from build123d import *

# Parameters (mm, degrees)
SKETCH_1_W          = 20
SKETCH_1_H          = 32.8
EXTRUDE_1_DEPTH     = 4
CUT_EXTRUDE_1_DEPTH = 1.6
SKETCH_4_R          = 2
CUT_EXTRUDE_2_DEPTH = 1.5
SKETCH_4_3_R        = 1.25
CUT_EXTRUDE_3_DEPTH = 39.624344655
SKETCH_5_W          = 20
SKETCH_5_H          = 6.2
EXTRUDE_4_DEPTH     = 2
EXTRUDE_START       = 2
SKETCH_5_6_W        = 20
SKETCH_5_6_H        = 4
EXTRUDE_5_DEPTH     = 5
SKETCH_6_R          = 1.25
CUT_EXTRUDE_4_DEPTH = 39.913750783
SKETCH_6_3_R        = 2
CUT_EXTRUDE_5_DEPTH = 1.5


with BuildPart() as part:
    # 草图1 → 凸台-拉伸1 (new body)
    with BuildSketch(Plane(origin=(0, 0, 0), x_dir=(1, 0, 0), z_dir=(0, 1, 0))):
        with Locations((10, -16.4)):
            Rectangle(SKETCH_1_W, SKETCH_1_H)
    extrude(amount=EXTRUDE_1_DEPTH)

    # 草图3 → 切除-拉伸1 (cut)
    with BuildSketch(Plane(origin=(0, 4, 0), x_dir=(-1, 0, 0), z_dir=(0, 1, 0))):
        with BuildLine():
            Line((-12.8, 13.543428629), (-12.095952788, 2.219685343))
            ThreePointArc((-12.095952788, 2.219685343), (-10, 0.25), (-7.904047212, 2.219685343))
            Line((-7.904047212, 2.219685343), (-7.2, 13.543428629))
            ThreePointArc((-7.2, 13.543428629), (-6, 16.4), (-7.2, 19.256571371))
            Line((-7.2, 19.256571371), (-7.904047212, 30.580314657))
            ThreePointArc((-7.904047212, 30.580314657), (-10, 32.55), (-12.095952788, 30.580314657))
            Line((-12.095952788, 30.580314657), (-12.8, 19.256571371))
            ThreePointArc((-12.8, 19.256571371), (-14, 16.4), (-12.8, 13.543428629))
        make_face()
    extrude(amount=-CUT_EXTRUDE_1_DEPTH, mode=Mode.SUBTRACT)

    # 草图4 → 切除-拉伸2 (cut)
    with BuildSketch(Plane.XZ):
        with Locations(Location((4, 4, 0), (0, 0, 270))):
            Circle(SKETCH_4_R)
        with Locations(Location((4, 28.8, 0), (0, 0, 270))):
            Circle(SKETCH_4_R)
        with Locations(Location((16, 28.8, 0), (0, 0, 270))):
            Circle(SKETCH_4_R)
        with Locations(Location((16, 4, 0), (0, 0, 270))):
            Circle(SKETCH_4_R)
    extrude(amount=-CUT_EXTRUDE_2_DEPTH, mode=Mode.SUBTRACT)

    # 草图4<3> → 切除-拉伸3 (cut, through all)
    with BuildSketch(Plane.XZ):
        with Locations(Location((4, 4, 0), (0, 0, 270))):
            Circle(SKETCH_4_3_R)
        with Locations(Location((4, 28.8, 0), (0, 0, 270))):
            Circle(SKETCH_4_3_R)
        with Locations(Location((16, 4, 0), (0, 0, 270))):
            Circle(SKETCH_4_3_R)
        with Locations(Location((16, 28.8, 0), (0, 0, 270))):
            Circle(SKETCH_4_3_R)
    extrude(amount=-CUT_EXTRUDE_3_DEPTH, mode=Mode.SUBTRACT)

    # 草图5 → 凸台-拉伸4 (add)
    with BuildSketch(Plane(origin=(0, 0, 0), x_dir=(-1, 0, 0), z_dir=(0, 0, -1))):
        with Locations((-10, 3.1)):
            Rectangle(SKETCH_5_W, SKETCH_5_H)
    extrude(amount=EXTRUDE_4_DEPTH)

    # 草图5<6> → 凸台-拉伸5 (add)
    with BuildSketch(Plane(origin=(0, 0, 0), x_dir=(-1, 0, 0), z_dir=(0, 0, -1)).offset(EXTRUDE_START)):
        with Locations((-10, 2)):
            Rectangle(SKETCH_5_6_W, SKETCH_5_6_H)
    extrude(amount=EXTRUDE_5_DEPTH)

    # 草图6 → 切除-拉伸4 (cut, through all)
    with BuildSketch(Plane.XZ):
        with Locations(Location((4, -4.5, 0), (0, 0, 270))):
            Circle(SKETCH_6_R)
        with Locations(Location((16, -4.5, 0), (0, 0, 270))):
            Circle(SKETCH_6_R)
    extrude(amount=-CUT_EXTRUDE_4_DEPTH, mode=Mode.SUBTRACT)

    # 草图6<3> → 切除-拉伸5 (cut)
    with BuildSketch(Plane.XZ):
        with Locations(Location((4, -4.5, 0), (0, 0, 270))):
            Circle(SKETCH_6_3_R)
        with Locations(Location((16, -4.5, 0), (0, 0, 270))):
            Circle(SKETCH_6_3_R)
    extrude(amount=-CUT_EXTRUDE_5_DEPTH, mode=Mode.SUBTRACT)


solid = part.part
Check sheet for the modelled part. Datum: model origin and axes. Units: mm. A direction names the side the tool comes from. Round coordinates to 2 decimals unless told otherwise and drop trailing zeros. Order: outer loops, then holes, each group sorted by start corner. A loop starts at its lowest first (then second) coordinate and runs counter-clockwise, first axis right, second up.
Q1. Cross-section at D-D, the plane x = 10. Enter the section's corners in (y, z).
Filled sheet:
outline: (0, -7) - (4, -7) - (4, -2) - (6.2, -2) - (6.2, 0) - (4, 0) - (4, 0.25) - (2.4, 0.25) - (2.4, 32.55) - (4, 32.55) - (4, 32.8) - (0, 32.8) - close
Q2. Cross-section at A-A, the plane x = 16. Give the number of separate pieces and of enclosed holes in the cut face, plus the area to 3 significant figures.
Filled sheet:
separate pieces: 4
enclosed holes: 0
area: 127 mm2
Q3. Cross-section at C-C, the plane y = 3. Enter the section's corners in (x, z), plus the area to 3 significant figures.
Filled sheet:
outline: (0, -7) - (20, -7) - (20, 32.8) - (0, 32.8) - close; hole circle Ø2.5 at (4, -4.5); hole circle Ø2.5 at (4, 4); hole circle Ø2.5 at (4, 28.8); hole (7.2, 13.54) - (7.9, 2.22) arc R2.1 ccw to (12.1, 2.22) - (12.8, 13.54) arc R4 ccw to (12.8, 19.26) - (12.1, 30.58) arc R2.1 ccw to (7.9, 30.58) - (7.2, 19.26) arc R4 ccw to start; hole circle Ø2.5 at (16, -4.5); hole circle Ø2.5 at (16, 4); hole circle Ø2.5 at (16, 28.8)
area: 601 mm2
Q4. Scan lines: L1, parallel to X at y = 0.6, z = 28.8; L2, parallel to Z at x = 3.75, y = 3; L3, parallel to Z at x = 16.5, y = 2. Record each from-to range of solid material in increasing order.
Filled sheet:
L1: x = 0 to 2, 6 to 14, 18 to 20
L2: z = -7 to -5.72, -3.28 to 2.78, 5.22 to 27.58, 30.02 to 32.8
L3: z = -7 to -5.65, -3.35 to 2.85, 5.15 to 27.65, 29.95 to 32.8
Q5. Depth check by flat-ended pin: P1, Ø6.5, axis at x = 16, z = 28.8, coming from the +Y side; P2, Ø3.5, axis at x = 4, z = 28.8, coming from the -Y side; P3, Ø2, axis at x = 10.5, z = 12.5, coming from the +Y side. Enter the tip coordinate at first touch or a pass-through.
Filled sheet:
P1: stops at y = 4
P2: stops at y = 1.5
P3: stops at y = 2.4
Q6. Set-up check for faces 5 (the face through (18, 1, 4)), 6 (the face through (10, 5, 0)), 7 (the face through (9.96, 3.21, 32.55)), 8 (the face through (2.78, 2.73, -4.23)): record each of +Z, -Z, +X, -X, +Y, -Y from which the full face is reachable in a straight line by a thin tool's end or side.
Filled sheet:
face 5: -Y
face 6: +Z, +X, -X, +Y
face 7: +Y
face 8: +Y, -Y
Q7. Cross-section at B-B, the plane z = -4.5. Enter the section's corners in (x, y).
Filled sheet:
outline: (0, 0) - (2, 0) - (2, 1.5) - (2.75, 1.5) - (2.75, 4) - (0, 4) - close; (5.25, 1.5) - (6, 1.5) - (6, 0) - (14, 0) - (14, 1.5) - (14.75, 1.5) - (14.75, 4) - (5.25, 4) - close; (17.25, 1.5) - (18, 1.5) - (18, 0) - (20, 0) - (20, 4) - (17.25, 4) - close
Q8. Draft check along Z on faces 1 (the face through (2.8, 0.7, 5.6)), 2 (the face through (20, 2, 13)), 3 (the face through (10, 2, -7)), 4 (the face through (14, 3.2, 16.4)). Enter one of: pulls with the +Z half, pulls with the -Z half, needs draft (parallel to the pull), parting line crosses it, or undercut.
Filled sheet:
face 1: undercut
face 2: needs draft
face 3: pulls with the -Z half
face 4: undercut
